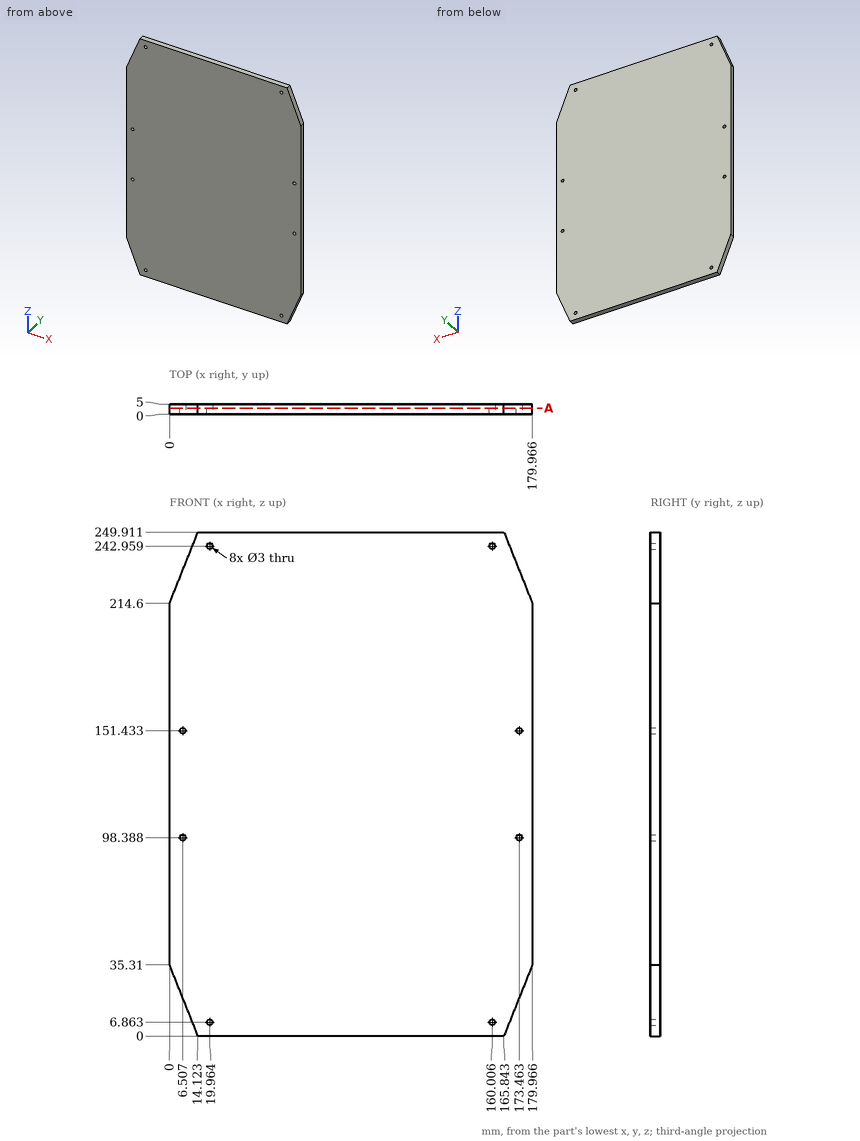
Can you work these out from the drawing? Everything is in mm from the part's minimum corner. Round coordinates to 2 decimals unless told otherwise and drop trailing zeros. Put each result on its own line as item: value.
Q1. For pin 1 Ø5 at (x, z) = (6.51, 98.39) entering from +Y, with a flat end and sliding along its axis, tell me the tip position at first contact or that it passes through.
Checks:
pin 1: y = 5
Q2. I want a section at A-A on y = 2.95. Give the number of separate pieces and of enclosed holes in the cut face, and give its area (3 significant figures).
Checks:
separate pieces: 1
enclosed holes: 8
area: 43,900 mm2
Q3. Please list where these lines run through material, in increasing order: line 1 (X direction, y = 2.9, z = 99) (1 decimal); line 2 (X direction, y = 1.45, z = 31.5) (1 decimal); line 3 (X direction, y = 3.95, z = 224) (1 decimal). Write a range as from..to.
Checks:
line 1: 0..5.1, 7.9..172.1, 174.8..180
line 2: 1.5..178.4
line 3: 3.8..176.2
